The listing builds one solid part. Answer for the finished solid, in the listing's coordinates (mm). Face numbers are marked on the shaded views. Coordinates: 2 decimals unless noted, no trailing zeros. Order: outer loops, then holes, each group sorted by start corner. A loop starts at its lowest first (then second) coordinate and runs counter-clockwise, first axis right, second up. Notation, with made-up numbers: (-20.75, -21) - (5.25, -21) arc R7 ccw to (5.25, -16) - close; hole circle Ø7 at (86, 14). An arc over 180 degrees is marked (long way). One line per item, written item: value. Start each with the question number.
```python
from build123d import *

# Parameters (mm, degrees)
F0_W     = 134.359292686
F0_H     = 65.8905915916
F1_DEPTH = 12.7
F2_W     = 134.359292686
F2_H     = 65.8905915916
F2_R     = 19.5560536298
F3_DEPTH = 151.7965264


# Not quite as in the source:
# - an extrude ends at something that could not be found from the text; its depth is read off the source's solid


with BuildPart() as f1:
    # F0 (on Top) → F1 (new body, symmetric)
    with BuildSketch(Plane.XY):
        with Locations((-0.1394487917, 6.2752943486)):
            Rectangle(F0_W, F0_H)
    extrude(amount=F1_DEPTH, both=True)

    # F2 (on face) → F3 (join, through all)
    with BuildSketch(Plane.XY.offset(12.7)):
        with Locations((-0.1394487917, 6.2752943486)):
            Rectangle(F2_W, F2_H)
        with Locations((-5.4052090272, 6.3866404817)):
            Circle(F2_R, mode=Mode.SUBTRACT)
    extrude(amount=F3_DEPTH)


solid = f1.part
```
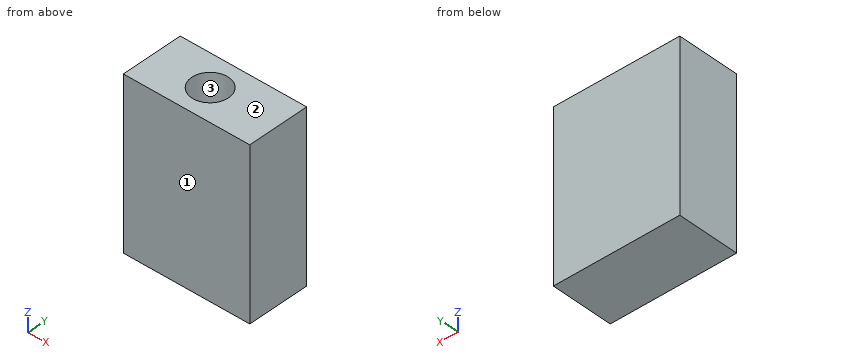
(1) Consider probe 1 along Y at (x, z) = (-5, 18); probe 2 along Y at (x, z) = (1, 92.5); probe 3 along X at (y, z) = (3, 47). Determine where each line is inside the solid, lowest interval first.
(2) The part is cut by section B-B on x = -12. Determine the outline of the cut face in (y, z).
(3) The part is cut by section C-C on y = 20.5. Determine the outline of the cut face in (x, z).
(4) For a pull along Y with two mould halves and no side action, classify the marked faces 1, 2 and 3 as pulls with the +Y half, pulls with the -Y half, needs draft (parallel to the pull), parting line crosses it, or undercut.
(5) The part is cut by section A-A on z = 140.5. Determine the outline of the cut face in (x, y).
Completed:
1. probe 1: y = -26.67 to -13.17, 25.94 to 39.22
1. probe 2: y = -26.67 to -12.09, 24.86 to 39.22
1. probe 3: x = -67.32 to -24.67, 13.86 to 67.04
2. outline: (-26.67, -12.7) - (39.22, -12.7) - (39.22, 164.5) - (24.8, 164.5) - (24.8, 12.7) - (-12.02, 12.7) - (-12.02, 164.5) - (-26.67, 164.5) - close
3. outline: (-67.32, -12.7) - (67.04, -12.7) - (67.04, 164.5) - (8.13, 164.5) - (8.13, 12.7) - (-18.94, 12.7) - (-18.94, 164.5) - (-67.32, 164.5) - close
4. face 1: pulls with the -Y half
4. face 2: needs draft
4. face 3: undercut
5. outline: (-67.32, -26.67) - (67.04, -26.67) - (67.04, 39.22) - (-67.32, 39.22) - close; hole circle Ø39.11 at (-5.41, 6.39)
